Could you check a few things on this drawing? It's one solid part, dimensions in mm from its lowest x, y, z. A direction names the side the tool comes from. Give positions to 0.01 mm unless a question says otherwise; leave off trailing zeros. Write each loop counter-clockwise with the first axis right and the second up, starting at its lowest first coordinate (ties: lowest second). Pieces come first, ordered by that corner, then holes. Notation, with made-up numbers: (86.25, 43.5) -> (134.25, 43.5) arc R15 cw to (134.25, 72.5) -> close; hole circle Ø3 at (74.25, 21.5). An arc over 180 degrees is marked (long way). Answer as CSV lines item,"result". Start each with the question number.
1. I need wall thicknesses on line 1 (Z direction, x = 29.75, y = 1.2); line 2 (Y direction, x = 13.5, z = 5.5). Which ranges of each line are inside material? Lowest first, please. Write a range as [from, to].
2. I'm going to push flat-ended pins straight in: P1, Ø5, axis at y = 5.5, z = 9, coming from the -X side; P2, Ø1.8, axis at x = 13.5, y = 5.5, coming from the +Z side; P3, Ø3, axis at y = 3.5, z = 14.5, coming from the +X side; P4, Ø2, axis at x = 26, y = 4, coming from the -Z side. Where does each tip first touch, or does it pass through?
3. On a 3-axis mill with a long thin cutter (end or side, diameter ignored), from which of +Z, -Z, +X, -X, +Y, -Y can I reach the whole of each face in a straight line? I mean the marked faces 1, 2, 3 and 4. Say none if no direction works.
4. If we section it at C-C on x = 16: Write out the boundary of the cut face in (y, z).
5. If we section it at D-D on y = 3.25: Write out the boundary of the cut face in (x, z).
6. If we section it at B-B on z = 2.25: Write out the boundary of the cut face in (x, y).
7. If we section it at A-A on x = 2.25: Write out the boundary of the cut face in (y, z).
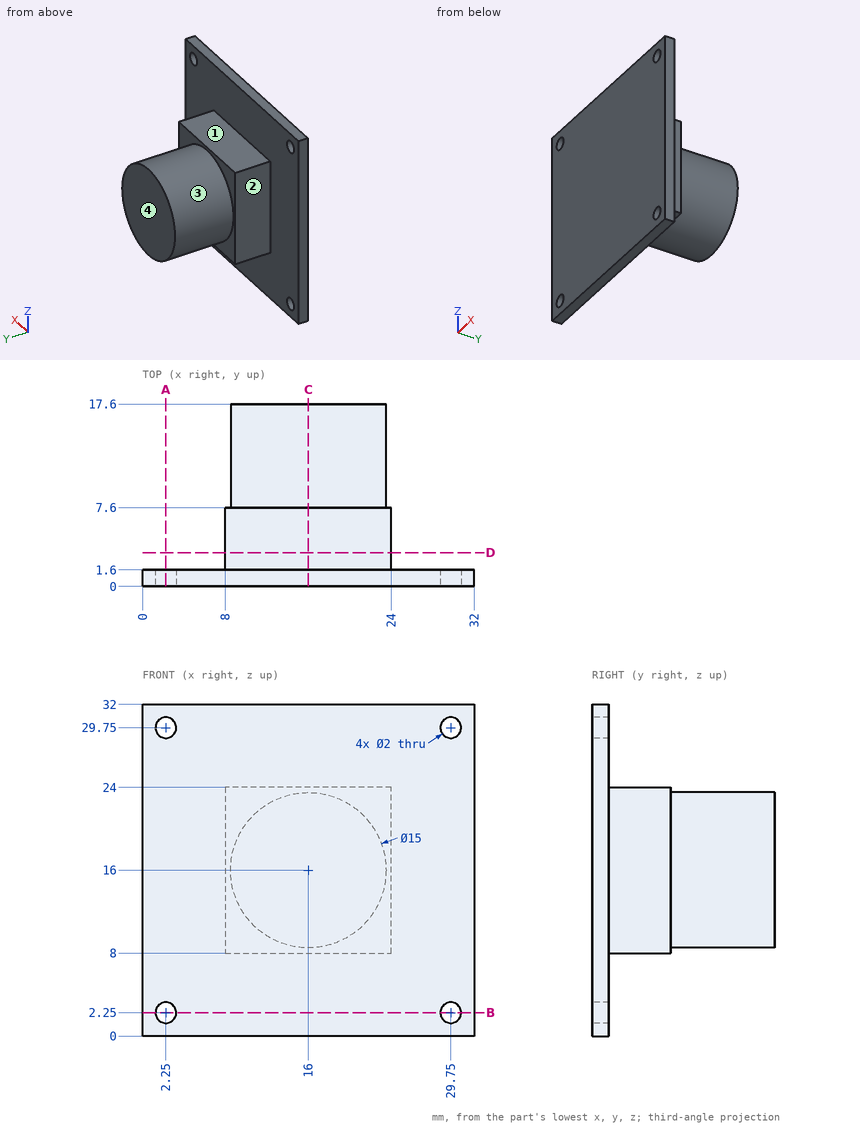
Computed values:
1,line 1,"z = [0, 1.25], [3.25, 28.75], [30.75, 32]"
1,line 2,"y = [0, 1.6]"
2,P1,"stops at x = 8"
2,P2,"stops at z = 24"
2,P3,"stops at x = 24"
2,P4,"passes through"
3,face 1,"+Z, +X, -X, +Y"
3,face 2,"+Z, -Z, -X, +Y"
3,face 3,"+Y"
3,face 4,"+Z, -Z, +X, -X, +Y"
4,outline,"(0, 0) -> (1.6, 0) -> (1.6, 8) -> (7.6, 8) -> (7.6, 8.5) -> (17.6, 8.5) -> (17.6, 23.5) -> (7.6, 23.5) -> (7.6, 24) -> (1.6, 24) -> (1.6, 32) -> (0, 32) -> close"
5,outline,"(8, 8) -> (24, 8) -> (24, 24) -> (8, 24) -> close"
6,outline,"(0, 0) -> (1.25, 0) -> (1.25, 1.6) -> (0, 1.6) -> close; (3.25, 0) -> (28.75, 0) -> (28.75, 1.6) -> (3.25, 1.6) -> close; (30.75, 0) -> (32, 0) -> (32, 1.6) -> (30.75, 1.6) -> close"
7,outline,"(0, 0) -> (1.6, 0) -> (1.6, 1.25) -> (0, 1.25) -> close; (0, 3.25) -> (1.6, 3.25) -> (1.6, 28.75) -> (0, 28.75) -> close; (0, 30.75) -> (1.6, 30.75) -> (1.6, 32) -> (0, 32) -> close"
